Here's how the part is built. I have some questions about the finished solid (model axes, mm). Give positions to 0.01 mm unless a question says otherwise; leave off trailing zeros. Loops run counter-clockwise (first coordinate to the right, second up) from the corner with the lowest first, then second, coordinate; pieces in that order, holes last. Notation, with made-up numbers: (40.25, 82.5) - (50.25, 82.5) arc R11 ccw to (50.25, 86.5) - close; hole circle Ø7 at (43.5, 78). An arc over 180 degrees is marked (long way). Use a Markdown table: item, result.
from build123d import *

# Parameters (mm, degrees)
EXTRUDE_1_DEPTH     = 270
SKETCH_2_R          = 2
CUT_EXTRUDE_1_DEPTH = 4
SKETCH_5_R          = 1.5
CUT_EXTRUDE_2_DEPTH = 4


with BuildPart() as part:
    # Эскиз1 → Бобышка-Вытянуть1 (new body)
    with BuildSketch(Plane(origin=(0, 0, 0), x_dir=(0, 0, -1), z_dir=(1, 0, 0))):
        Polygon((0, 0), (-10, 0), (-10, 3), (-3, 3), (-3, 10), (0, 10), align=None)
    extrude(amount=EXTRUDE_1_DEPTH)

    # Эскиз2 → Вырез-Вытянуть1 (cut, through all)
    with BuildSketch(Plane.XY.offset(3)):
        with Locations((25, 6.5)):
            Circle(SKETCH_2_R)
        with Locations((245, 6.5)):
            Circle(SKETCH_2_R)
    extrude(amount=-CUT_EXTRUDE_1_DEPTH, mode=Mode.SUBTRACT)

    # Эскиз5 → Вырез-Вытянуть2 (cut, through all)
    with BuildSketch(Plane.XY.offset(3)):
        with Locations((8, 6.5)):
            Circle(SKETCH_5_R)
        with Locations((262, 6.5)):
            Circle(SKETCH_5_R)
    extrude(amount=-CUT_EXTRUDE_2_DEPTH, mode=Mode.SUBTRACT)


solid = part.part
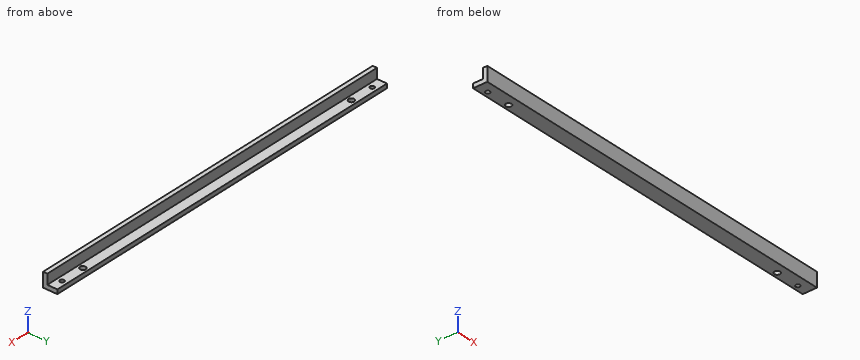
(1) Suppose I cut it at C-C on z = 6. Write out the boundary of the cut face in (x, y), plus the area to 3 significant figures.
A:
| item | result |
|---|---|
| outline | (0, 0) - (270, 0) - (270, 3) - (0, 3) - close |
| area | 810 mm2 |
(2) Suppose I cut it at A-A on y = 6.5. Write out the boundary of the cut face in (x, z).
A:
| item | result |
|---|---|
| outline | (0, 0) - (6.5, 0) - (6.5, 3) - (0, 3) - close; (9.5, 0) - (23, 0) - (23, 3) - (9.5, 3) - close; (27, 0) - (243, 0) - (243, 3) - (27, 3) - close; (247, 0) - (260.5, 0) - (260.5, 3) - (247, 3) - close; (263.5, 0) - (270, 0) - (270, 3) - (263.5, 3) - close |
(3) Will these pins go through, and if not, where does the flat tip stop? pin 1 (5 mm diameter, centred on x = 262, y = 6.5, fed in from +Z); pin 2 (2 mm diameter, centred on x = 195.5, z = 7.5, fed in from +Y).
A:
| item | result |
|---|---|
| pin 1 | z = 3 |
| pin 2 | y = 3 |
(4) Suppose I cut it at B-B on x = 176. Write out the boundary of the cut face in (y, z).
A:
| item | result |
|---|---|
| outline | (0, 0) - (10, 0) - (10, 3) - (3, 3) - (3, 10) - (0, 10) - close |
(5) If I drill on line 1 (Y direction, x = 262, z = 1.35); line 2 (Y direction, x = 25, z = 2.25); line 3 (Y direction, x = 47.5, z = 8.5), over which ranges is the centre line in solid material (lowest first)?
A:
| item | result |
|---|---|
| line 1 | 0 to 5, 8 to 10 |
| line 2 | 0 to 4.5, 8.5 to 10 |
| line 3 | 0 to 3 |
